Input: part model. Units: mm. Frame: model coordinates. A direction names the side the tool comes from. Give positions to 0.01 mm unless a question says otherwise; leave off trailing zeros. Order: outer loops, then holes, each group sorted by start corner. A loop starts at its lowest first (then second) coordinate and runs counter-clockwise, first axis right, second up. Notation, with made-up numbers: (-10.5, -25.5) - (24.5, -25.5) arc R25 ccw to (24.5, 6.5) - close; hole circle Ø5 at (-26.75, -32.75). An arc over 180 degrees is marked (long way). Answer in a Markdown table with one row per item. Add a question column.
from build123d import *

# Parameters (mm, degrees)
F1_DEPTH = 2
F3_DEPTH = 2
F5_DEPTH = 1


with BuildPart() as f1:
    # F0 (on Top) → F1 (new body)
    with BuildSketch(Plane.XY):
        with BuildLine():
            Line((-1.1952485209, 11.4377174722), (-1.3927243635, 13.3274273154))
            ThreePointArc((-1.3927243635, 13.3274273154), (-2.5775676265, 13.1497583678), (-3.7418055675, 12.8669689941))
            Line((-3.7418055675, 12.8669689941), (-3.2112510467, 11.0425480173))
            ThreePointArc((-3.2112510467, 11.0425480173), (-2.2120916198, 11.2852403902), (-1.1952485209, 11.4377174722))
        make_face()
        with BuildLine():
            Line((-1.3927243635, 13.3274273154), (-1.5590198098, 14.9187619202))
            ThreePointArc((-1.5590198098, 14.9187619202), (-15, 0), (-1.5590198098, -14.9187619202))
            Line((-1.5590198098, -14.9187619202), (-1.3927243635, -13.3274273154))
            ThreePointArc((-1.3927243635, -13.3274273154), (-13.3464395592, -1.1968922642), (-3.7418055675, 12.8669689941))
            ThreePointArc((-3.7418055675, 12.8669689941), (-2.5775676265, 13.1497583678), (-1.3927243635, 13.3274273154))
        make_face()
    extrude(amount=F1_DEPTH)

    # F2 (on face) → F3, piece 2 (join)
    with BuildSketch(Plane.XY.offset(2)):
        with BuildLine():
            ThreePointArc((-4.1885883218, 14.4033235009), (-14.9400442827, -1.3398047734), (-1.5590198098, -14.9187619202))
            Line((-1.5590198098, -14.9187619202), (-1.3927243635, -13.3274273154))
            ThreePointArc((-1.3927243635, -13.3274273154), (-13.3464395592, -1.1968922642), (-3.7418055675, 12.8669689941))
            Line((-3.7418055675, 12.8669689941), (-4.1885883218, 14.4033235009))
        make_face()
    extrude(amount=F3_DEPTH)



with BuildPart() as f1b:
    # F0 (on Top) → F1, piece 2 (new body)
    with BuildSketch(Plane.XY):
        with BuildLine():
            ThreePointArc((1.5731137528, -14.9172823638), (11.1489171289, -10.0350210191), (15, 0))
            ThreePointArc((15, 0), (11.1489171289, 10.0350210191), (1.5731137528, 14.9172823638))
            Line((1.5731137528, 14.9172823638), (1.3927243635, 13.3274273154))
            ThreePointArc((1.3927243635, 13.3274273154), (9.9554634867, 8.9693225366), (13.4, 0))
            ThreePointArc((13.4, 0), (10.7168137663, -8.0442465587), (3.7418055675, -12.8669689941))
            ThreePointArc((3.7418055675, -12.8669689941), (2.5775676265, -13.1497583678), (1.3927243635, -13.3274273154))
            Line((1.3927243635, -13.3274273154), (1.5731137528, -14.9172823638))
        make_face()
        with BuildLine():
            Line((1.1952485209, -11.4377174722), (1.3927243635, -13.3274273154))
            ThreePointArc((1.3927243635, -13.3274273154), (2.5775676265, -13.1497583678), (3.7418055675, -12.8669689941))
            Line((3.7418055675, -12.8669689941), (3.2112510467, -11.0425480173))
            ThreePointArc((3.2112510467, -11.0425480173), (2.2120916198, -11.2852403902), (1.1952485209, -11.4377174722))
        make_face()
    extrude(amount=F1_DEPTH)

    # F2 (on face) → F3 (join)
    with BuildSketch(Plane.XY.offset(2)):
        with BuildLine():
            ThreePointArc((4.1885883218, -14.4033235009), (11.9964333205, -9.0047536105), (15, 0))
            ThreePointArc((15, 0), (11.1441755448, 10.0402864215), (1.5590198098, 14.9187619202))
            Line((1.5590198098, 14.9187619202), (1.3927243635, 13.3274273154))
            ThreePointArc((1.3927243635, 13.3274273154), (9.9554634867, 8.9693225366), (13.4, 0))
            ThreePointArc((13.4, 0), (10.7168137663, -8.0442465587), (3.7418055675, -12.8669689941))
            Line((3.7418055675, -12.8669689941), (4.1885883218, -14.4033235009))
        make_face()
    extrude(amount=F3_DEPTH)


with BuildPart() as f1_1:
    add(f1.part)

    add(f1b.part)  # F5 merges F1b
    # F4 (on face) → F5 (join)
    with BuildSketch(Plane.XY.offset(4)):
        with BuildLine():
            Line((-3.7418055675, 12.8669689941), (-4.1885883218, 14.4033235009))
            ThreePointArc((-4.1885883218, 14.4033235009), (-14.9400442827, -1.3398047734), (-1.5590198098, -14.9187619202))
            Line((-1.5590198098, -14.9187619202), (-1.3927243635, -13.3274273154))
            ThreePointArc((-1.3927243635, -13.3274273154), (-13.3464395592, -1.1968922642), (-3.7418055675, 12.8669689941))
        make_face()
        with BuildLine():
            ThreePointArc((-1.5590198098, -14.9187619202), (10.0402864215, -11.1441755448), (15, 0))
            ThreePointArc((15, 0), (9.0047536105, 11.9964333205), (-4.1885883218, 14.4033235009))
            Line((-4.1885883218, 14.4033235009), (-3.7418055675, 12.8669689941))
            ThreePointArc((-3.7418055675, 12.8669689941), (8.0442465587, 10.7168137663), (13.4, 0))
            ThreePointArc((13.4, 0), (8.9693225366, -9.9554634867), (-1.3927243635, -13.3274273154))
            Line((-1.3927243635, -13.3274273154), (-1.5590198098, -14.9187619202))
        make_face()
    extrude(amount=F5_DEPTH)


solid = f1_1.part
Q1. Section B-B, the plane x = 0. Return loops of the section in (y, z).
Q2. Pull-direction query (Z, two-part tool) for faces 1 (the flat face through (-14, 1, 0)), 2 (the flat face through (-3, 13, 2)), 3 (the cylindrical face through (2.23, -11.28, 0.99)); classes: +Z half, -Z half, draft (parallel to the pull), parting line (faces both ways), or undercut.
Q3. Line query: probe 1 along Y at (x, z) = (8, 2.6); probe 2 along X at (y, z) = (0.25, 0.3); probe 3 along Y at (x, z) = (-4, 0.7). Output: solid intervals per line, ascending.
Q4. Access query for faces 4 (the flat face through (-3.48, 11.97, 0.99)), 5 (the flat face through (3.96, -13.62, 2.99)), 6 (the flat face through (-1, 14, 4)). Directions: +Z, -Z, +X, -X, +Y, -Y. A direction counts if a zero-diameter tool reaches every point of the face in a straight line with its end or side. Return the directions, or none.
Q5. Contact query for flat-ended pins moving along their axis: P1, Ø6, axis at x = 7.5, y = 10.5, coming from the -Z side; P2, Ø2, axis at x = -6.5, z = 1, coming from the -Y side; P3, Ø1, axis at x = -9.5, z = 0.5, coming from the -Y side; P4, Ø1, axis at x = -2, z = 1, coming from the -Y side. Output: stop coordinate, or through.
Q6. Section C-C, the plane y = -9.5. Return loops of the section in (x, z), then the cut area to 3 significant figures.
Q7. Section D-D, the plane z = 0.8. Return loops of the section in (x, y).
Q8. Section A-A, the plane z = 3.2. Return loops of the section in (x, y).
Computed:
| question | item | result |
|---|---|---|
| 1 | outline | (-15, 4) - (-13.4, 4) - (-13.4, 5) - (-15, 5) - close; (13.4, 4) - (15, 4) - (15, 5) - (13.4, 5) - close |
| 2 | face 1 | -Z half |
| 2 | face 2 | undercut |
| 2 | face 3 | draft |
| 3 | probe 1 | y = -12.69 to -10.75, 10.75 to 12.69 |
| 3 | probe 2 | x = -15 to -13.4, 13.4 to 15 |
| 3 | probe 3 | y = -14.46 to -12.79, 12.79 to 14.46 |
| 4 | face 4 | +Z, -Z |
| 4 | face 5 | -Y |
| 4 | face 6 | +Y |
| 5 | P1 | stops at z = 0 |
| 5 | P2 | stops at y = -13.96 |
| 5 | P3 | stops at y = -12 |
| 5 | P4 | stops at y = -14.92 |
| 6 | outline | (-11.61, 0) - (-9.45, 0) - (-9.45, 5) - (-11.61, 5) - close; (9.45, 0) - (11.61, 0) - (11.61, 5) - (9.45, 5) - close |
| 6 | area | 21.6 mm^2 |
| 7 | outline | (-3.74, 12.87) - (-3.21, 11.04) arc R11.5 cw to (-1.2, 11.44) - (-1.56, 14.92) arc R15 ccw to (-1.56, -14.92) - (-1.39, -13.33) arc R13.4 cw to start; (1.2, -11.44) - (1.39, -13.33) - (1.57, -14.92) arc R15 ccw to (1.57, 14.92) - (1.39, 13.33) arc R13.4 cw to (3.74, -12.87) - (3.21, -11.04) arc R11.5 cw to start |
| 8 | outline | (-4.19, 14.4) arc R15 ccw to (-1.56, -14.92) - (-1.39, -13.33) arc R13.4 cw to (-3.74, 12.87) - close; (1.39, 13.33) arc R13.4 cw to (3.74, -12.87) - (4.19, -14.4) arc R15 ccw to (1.56, 14.92) - close |
